```python
from build123d import *

# Parameters (mm, degrees)
F1_DEPTH      = 0.762
F2_R          = 2.54
F3_R          = 0.508
F4_R          = 3.0139316414
F5_DEPTH      = 0.254
F6_R          = 1.524
F7_DEPTH      = 1.27
F8_SIZE       = 0.254
F9_R          = 0.381
F10_DEPTH     = 0.254
F11_R         = 1.016
F12_DEPTH     = 25.4
F13_R         = 0.25399
F15_DEPTH     = 0.508
F16_T1_DEPTH  = 7.366
F16_T3_DEPTH  = 7.366
F16_T6_ANGLE  = 180
F16_T8_ANGLE  = 180
F16_T10_ANGLE = 180
F16_T12_ANGLE = 180


# Not quite as in the source:
# - a fillet or chamfer that OpenCascade refuses, or shapes differently, is made with other operations: its cross-section is extruded or revolved along the edge and cut away or added
# - a fillet or chamfer is up to 0.001 mm smaller than in the source, because OpenCascade refuses the exact size


with BuildPart() as f1:
    # F0 (on Top) → F1 (new body)
    with BuildSketch(Plane.XY):
        with BuildLine():
            Line((2.032, -14.605), (2.032, -2.6027254946))
            ThreePointArc((2.032, -2.6027254946), (3.302, 0), (2.032, 2.6027254946))
            Line((2.032, 2.6027254946), (2.032, 14.605))
            Line((2.032, 14.605), (2.032, 22.225))
            Line((2.032, 22.225), (-2.032, 22.225))
            Line((-2.032, 22.225), (-2.032, 14.605))
            Line((-2.032, 14.605), (-2.032, 2.6027254946))
            ThreePointArc((-2.032, 2.6027254946), (-3.302, 0), (-2.032, -2.6027254946))
            Line((-2.032, -2.6027254946), (-2.032, -14.605))
            Line((-2.032, -14.605), (-2.032, -22.225))
            Line((-2.032, -22.225), (2.032, -22.225))
            Line((2.032, -22.225), (2.032, -14.605))
        make_face()
    extrude(amount=F1_DEPTH)

    # F2
    f2_edges = [f1.edges().sort_by_distance(p)[0] for p in [
        (-2.032, 2.602725, 0.381),
        (-2.032, -2.602725, 0.381),
        (2.032, 2.602725, 0.381),
        (2.032, -2.602725, 0.381),
    ]]
    fillet(f2_edges, radius=F2_R)

    # F3
    f3_edges = [f1.edges().sort_by_distance(p)[0] for p in [
        (-2.032, -22.225, 0.381),
        (2.032, -22.225, 0.381),
        (-2.032, 22.225, 0.381),
        (2.032, 22.225, 0.381),
    ]]
    fillet(f3_edges, radius=F3_R)

    # F4 (on face) → F5 (join)
    with BuildSketch(Plane.XY.offset(0.762)):
        Circle(F4_R)
    extrude(amount=F5_DEPTH)

    # F6 (on face) → F7 (join)
    with BuildSketch(Plane.XY.offset(1.016)):
        Circle(F6_R)
    extrude(amount=F7_DEPTH)

    # F8
    f8_edges = [f1.edges().sort_by_distance(p)[0] for p in [
        (-1.524, 0, 2.286),
    ]]
    chamfer(f8_edges, length=F8_SIZE)

    # F9 (on face) → F10 (join)
    with BuildSketch(Plane.XY.offset(1.016)):
        with Locations((0, 2.1844)):
            Circle(F9_R)
        with Locations((0, -2.1844)):
            Circle(F9_R)
    extrude(amount=F10_DEPTH)

    # F11 (on face) → F12 (cut)
    with BuildSketch(Plane.XY.offset(2.286)):
        Circle(F11_R)
    extrude(amount=-F12_DEPTH, mode=Mode.SUBTRACT)

    # F13 (radius 0.254 in the source; OpenCascade refuses exactly that, so slightly less here)
    f13_edges = [f1.edges().sort_by_distance(p)[0] for p in [
        (-1.016, 0, 2.286),
        (-1.016, 0, 0),
    ]]
    fillet(f13_edges, radius=F13_R)

    # F14 (on face) → F15 (join)
    with BuildSketch(Plane.XY.offset(0.762)):
        with BuildLine():
            ThreePointArc((0, 12.7), (-0.5388153673, 12.4768153673), (-0.762, 11.938))
            Line((-0.762, 11.938), (-0.762, 4.572))
            ThreePointArc((-0.762, 4.572), (-0.5388153673, 4.0331846327), (0, 3.81))
            ThreePointArc((0, 3.81), (0.5388153673, 4.0331846327), (0.762, 4.572))
            Line((0.762, 4.572), (0.762, 11.938))
            ThreePointArc((0.762, 11.938), (0.5388153673, 12.4768153673), (0, 12.7))
        make_face()
        with BuildLine():
            ThreePointArc((0, -3.81), (-0.5388153673, -4.0331846327), (-0.762, -4.572))
            Line((-0.762, -4.572), (-0.762, -11.938))
            ThreePointArc((-0.762, -11.938), (-0.5388153673, -12.4768153673), (0, -12.7))
            ThreePointArc((0, -12.7), (0.5388153673, -12.4768153673), (0.762, -11.938))
            Line((0.762, -11.938), (0.762, -4.572))
            ThreePointArc((0.762, -4.572), (0.5388153673, -4.0331846327), (0, -3.81))
        make_face()
    extrude(amount=F15_DEPTH)

    # F16: fillet of radius 0.762 on 8 edges, made by hand

    # F16_s2 → F16_t1 (cut)
    with BuildSketch(Plane.XZ.offset(-11.938)):
        with BuildLine():
            ThreePointArc((-0.762, 0.762), (-0.4835204154, 1.1301703947), (-0.0435795103, 1.27))
            Line((-0.0435795103, 1.27), (-0.762, 1.27))
            Line((-0.762, 1.27), (-0.762, 0.762))
        make_face()
        with BuildLine():
            ThreePointArc((0.762, 0.762), (0.4835204154, 1.1301703947), (0.0435795103, 1.27))
            Line((0.0435795103, 1.27), (0.762, 1.27))
            Line((0.762, 1.27), (0.762, 0.762))
        make_face()
    extrude(amount=F16_T1_DEPTH, mode=Mode.SUBTRACT)

    # F16_s4 → F16_t3 (cut)
    with BuildSketch(Plane.XZ.offset(4.572)):
        with BuildLine():
            ThreePointArc((-0.762, 0.762), (-0.4835204154, 1.1301703947), (-0.0435795103, 1.27))
            Line((-0.0435795103, 1.27), (-0.762, 1.27))
            Line((-0.762, 1.27), (-0.762, 0.762))
        make_face()
        with BuildLine():
            ThreePointArc((0.762, 0.762), (0.4835204154, 1.1301703947), (0.0435795103, 1.27))
            Line((0.0435795103, 1.27), (0.762, 1.27))
            Line((0.762, 1.27), (0.762, 0.762))
        make_face()
    extrude(amount=F16_T3_DEPTH, mode=Mode.SUBTRACT)

    # F16_s5 → F16_t6 (revolve, cut)
    with BuildSketch(Plane.XZ.offset(-11.938)):
        with BuildLine():
            ThreePointArc((0.762, 0.762), (0.4835204154, 1.1301703947), (0.0435795103, 1.27))
            Line((0.0435795103, 1.27), (0.762, 1.27))
            Line((0.762, 1.27), (0.762, 0.762))
        make_face()
    revolve(axis=Axis((0, 11.938, 1.27), (0, 0, 1)), revolution_arc=F16_T6_ANGLE, mode=Mode.SUBTRACT)

    # F16_s7 → F16_t8 (revolve, cut)
    with BuildSketch(Plane.XZ.offset(-4.572)):
        with BuildLine():
            ThreePointArc((-0.762, 0.762), (-0.4835204154, 1.1301703947), (-0.0435795103, 1.27))
            Line((-0.0435795103, 1.27), (-0.762, 1.27))
            Line((-0.762, 1.27), (-0.762, 0.762))
        make_face()
    revolve(axis=Axis((0, 4.572, 1.27), (0, 0, 1)), revolution_arc=F16_T8_ANGLE, mode=Mode.SUBTRACT)

    # F16_s9 → F16_t10 (revolve, cut)
    with BuildSketch(Plane.XZ.offset(4.572)):
        with BuildLine():
            ThreePointArc((0.762, 0.762), (0.4835204154, 1.1301703947), (0.0435795103, 1.27))
            Line((0.0435795103, 1.27), (0.762, 1.27))
            Line((0.762, 1.27), (0.762, 0.762))
        make_face()
    revolve(axis=Axis((0, -4.572, 1.27), (0, 0, 1)), revolution_arc=F16_T10_ANGLE, mode=Mode.SUBTRACT)

    # F16_s11 → F16_t12 (revolve, cut)
    with BuildSketch(Plane.XZ.offset(11.938)):
        with BuildLine():
            ThreePointArc((-0.762, 0.762), (-0.4835204154, 1.1301703947), (-0.0435795103, 1.27))
            Line((-0.0435795103, 1.27), (-0.762, 1.27))
            Line((-0.762, 1.27), (-0.762, 0.762))
        make_face()
    revolve(axis=Axis((0, -11.938, 1.27), (0, 0, 1)), revolution_arc=F16_T12_ANGLE, mode=Mode.SUBTRACT)


solid = f1.part
```
Can you work these out from the model? Positions are in its coordinate system, mm. A direction names the side the tool comes from. Coordinates: 2 decimals unless noted, no trailing zeros. Write each loop counter-clockwise with the first axis right and the second up, starting at its lowest first coordinate (ties: lowest second). Pieces come first, ordered by that corner, then holes. Notation, with made-up numbers: M 66.25,59 L 85.25,59 A21 ccw 85.25,91 Z; hole C 47,-16.75 d3. An arc over 180 degrees is marked long. Write item = value, one per line. Start each with the question number.
Q1. Thinking about a two-plate mould opening in X: for faces 3 (the face through (-1, 5, 0.762)), 4 (the face through (-0.22, -0.99, 1.16)), 5 (the face through (-0.2, 1.51, 1.52)), which applies, released by +X, released by -X, zero draft, split by the parting line, or undercut?
Q2. I'm going to push flat-ended pins straight in: pin 1 (0.6 mm diameter, centred on x = 0, y = -2, fed in from +Z); pin 2 (0.6 mm diameter, centred on y = 16, z = 0.5, fed in from -X); pin 3 (0.6 mm diameter, centred on y = -8.5, z = 0.5, fed in from +X). Where does each tip first touch, or does it pass through?
Q3. If I drill on L1, parallel to Y at x = 0, z = 1.35; L2, parallel to Y at x = 0, z = 1.1; L3, parallel to Y at x = -0.5, z = 0.8, over which ranges is the centre line in solid material (lowest first)? Write a range as [from, to].
Q4. On a 3-axis mill with a long thin cutter (end or side, diameter ignored), from which of +Z, -Z, +X, -X, +Y, -Y can I reach the whole of each face in a straight line? I mean faces 1 (the face through (1.3, -1.3, 1.016)), 2 (the face through (1.4, 0.3, 0)). Say none if no direction works.
Q5. If we section it at B-B, the plane y = -10.5: Write out the boundary of the cut face in (x, z).
Q6. If we section it at C-C, the plane y = 16: Write out the boundary of the cut face in (x, z).
Check sheet entries:
q1.face_3 = zero draft
q1.face_4 = undercut
q1.face_5 = split by the parting line
q2.pin_1 = 1.27
q2.pin_2 = -2.03
q2.pin_3 = 2.03
q3.L1 = [-1.52, -1.02], [1.02, 1.52]
q3.L2 = [-12.46, -4.05], [-2.57, -1.8], [-1.52, -1.02], [1.02, 1.52], [1.8, 2.57], [4.05, 12.46]
q3.L3 = [-12.49, -4.02], [-2.97, -0.88], [0.88, 2.97], [4.02, 12.49]
q4.face_1 = +Z
q4.face_2 = -Z, +X, -X, +Y, -Y
q5.outline = M -2.03,0 L 2.03,0 L 2.03,0.76 L 0.76,0.76 A0.76 ccw 0.04,1.27 L -0.04,1.27 A0.76 ccw -0.76,0.76 L -2.03,0.76 Z
q6.outline = M -2.03,0 L 2.03,0 L 2.03,0.76 L -2.03,0.76 Z
